Geometry: final body of the model. Coordinates: model frame, mm. A direction names the side the tool comes from. Give positions to 0.01 mm unless a question says otherwise; leave off trailing zeros. Loops run counter-clockwise (first coordinate to the right, second up) from the corner with the lowest first, then second, coordinate; pieces in that order, holes last. Notation, with made-up numbers: (7, 39.5) -> (28, 39.5) arc R21 ccw to (28, 53.5) -> close; hole circle Ø3 at (-8, -19.5). An arc over 180 degrees is marked (long way). One line per question, with ' | ' between items. Start each with the question number.
Item 1: Section D-D on x = 262.5. Return loops of the section in (y, z).
Item 2: Section C-C on x = -12. Return loops of the section in (y, z).
Item 3: Material intervals for line 1 along Y through (x, z) = (-311.95, 6); line 2 along Z through (x, y) = (312, -68); line 3 along Z through (x, y) = (-81, -12), sorted ascending. Write a range as [from, to].
Item 4: Set-up query: faces 4 (the flat face through (-326.8, -4.6, 0)), 5 (the flat face through (2, -17, 103)), 6 (the flat face through (-322, -61, 0)). Return all of +Z, -Z, +X, -X, +Y, -Y with unobstructed straight access to the full face (end or side cutting, diameter ignored); none if empty.
Item 5: Section A-A on y = -79.5. Return loops of the section in (x, z).
Item 6: Pin query (flat end, axial travel): P1, Ø0.5, axis at x = -312, y = -60, coming from the +Z side; P2, Ø3, axis at x = 110.3, z = 6, coming from the -Y side; P3, Ø9, axis at x = 71, z = 5.5, coming from the -Y side. Return the tip coordinate at first contact, or that it passes through.
Item 7: Mould query, pull axis X, two halves, no side actions, for faces 1 (the flat face through (4, 1, 51)), 2 (the flat face through (-4, 0, 51)), 3 (the cylindrical face through (-326.889, -3.563, 51.272)). Classes: released by +X, released by -X, zero draft, split by the parting line, or undercut.
Item 8: Section B-B on z = 18. Return loops of the section in (x, y), then the cut area to 3 significant figures.
from build123d import *

# Parameters (mm, degrees)
BASE_FLANGE1_DEPTH             = 104
EDGE_FLANGE1_STRIP_W           = 6
EDGE_FLANGE1_STRIP_H           = 1
EDGE_FLANGE1_STRIP_CUT_DEPTH   = 621.4
EDGE_FLANGE1_RELIEF_W          = 6.5
EDGE_FLANGE1_RELIEF_H          = 0.5
EDGE_FLANGE1_RELIEF_CUT_DEPTH  = 1
EDGE_FLANGE1_DEPTH             = 621.4
EDGE_FLANGE2_STRIP_W           = 6
EDGE_FLANGE2_STRIP_H           = 1
EDGE_FLANGE2_STRIP_CUT_DEPTH   = 621.4
EDGE_FLANGE2_DEPTH             = 621.4
EDGE_FLANGE3_STRIP_W           = 6
EDGE_FLANGE3_STRIP_H           = 1
EDGE_FLANGE3_STRIP_CUT_DEPTH   = 80
EDGE_FLANGE3_RELIEF_W          = 6.5
EDGE_FLANGE3_RELIEF_H          = 0.5
EDGE_FLANGE3_RELIEF_CUT_DEPTH  = 1
EDGE_FLANGE3_DEPTH             = 80
EDGE_FLANGE4_STRIP_W           = 6
EDGE_FLANGE4_STRIP_H           = 1
EDGE_FLANGE4_STRIP_CUT_DEPTH   = 80
EDGE_FLANGE4_DEPTH             = 80
EDGE_FLANGE5_STRIP_W           = 6
EDGE_FLANGE5_STRIP_H           = 1
EDGE_FLANGE5_STRIP_CUT_DEPTH   = 221.4
EDGE_FLANGE5_RELIEF_W          = 6.5
EDGE_FLANGE5_RELIEF_H          = 0.5
EDGE_FLANGE5_RELIEF_CUT_DEPTH  = 1
EDGE_FLANGE5_DEPTH             = 221.4
SKETCH22_R                     = 2.5
CUT_EXTRUDE1_DEPTH             = 1
SKETCH23_R                     = 2.5
CUT_EXTRUDE2_DEPTH             = 3
CUT_EXTRUDE2_DIRECTION_2_REACH = 661.378
EDGE_FLANGE6_STRIP_W           = 6
EDGE_FLANGE6_STRIP_H           = 1
EDGE_FLANGE6_STRIP_CUT_DEPTH   = 221.4
EDGE_FLANGE6_DEPTH             = 221.4
EDGE_FLANGE6_FLAT_DEPTH        = 1


# Sheet-metal steps are written as plain solids
with BuildPart() as part:
    # Sketch1 → Base-Flange1 (new body)
    with BuildSketch(Plane.XY):
        with BuildLine():
            Line((-330.7, -100), (-330.7, -15))
            ThreePointArc((-330.7, -15), (-326.306601718, -4.393398282), (-315.7, 0))
            Line((-315.7, 0), (315.7, 0))
            ThreePointArc((315.7, 0), (326.306601718, -4.393398282), (330.7, -15))
            Line((330.7, -15), (330.7, -100))
            Line((330.7, -100), (331.7, -100))
            Line((331.7, -100), (331.7, -15))
            ThreePointArc((331.7, -15), (327.013708499, -3.686291501), (315.7, 1))
            Line((315.7, 1), (-315.7, 1))
            ThreePointArc((-315.7, 1), (-327.013708499, -3.686291501), (-331.7, -15))
            Line((-331.7, -15), (-331.7, -100))
            Line((-331.7, -100), (-330.7, -100))
        make_face()
    extrude(amount=BASE_FLANGE1_DEPTH)

    # Edge-Flange1 strip (across the edge) → Edge-Flange1 strip cut (cut)
    with BuildSketch(Plane(origin=(-310.7, 0, 0), x_dir=(0, 0, 1), z_dir=(1, 0, 0))):
        with Locations((-2, -0.5)):
            Rectangle(EDGE_FLANGE1_STRIP_W, EDGE_FLANGE1_STRIP_H)
    extrude(amount=EDGE_FLANGE1_STRIP_CUT_DEPTH, mode=Mode.SUBTRACT)

    # Edge-Flange1 relief (on the sheet) → Edge-Flange1 relief cut (cut)
    with BuildSketch(Plane(origin=(-310.7, 0, 1), x_dir=(0, 0, 1), z_dir=(0, -1, 0))):
        with Locations((-2.75, 0.25)):
            Rectangle(EDGE_FLANGE1_RELIEF_W, EDGE_FLANGE1_RELIEF_H)
        with Locations((-2.75, -621.65)):
            Rectangle(EDGE_FLANGE1_RELIEF_W, EDGE_FLANGE1_RELIEF_H)
    extrude(amount=-EDGE_FLANGE1_RELIEF_CUT_DEPTH, mode=Mode.SUBTRACT)

    # Edge-Flange1 section (across the edge) → Edge-Flange1 (add)
    with BuildSketch(Plane(origin=(-310.7, 0, 0), x_dir=(0, 0, 1), z_dir=(1, 0, 0))):
        with BuildLine():
            Line((-1, 1), (-1, 19))
            Line((-1, 19), (0, 19))
            Line((0, 19), (0, 1))
            ThreePointArc((0, 1), (0.292893219, 0.292893219), (1, 0))
            Line((1, 0), (1, -1))
            ThreePointArc((1, -1), (-0.414213562, -0.414213562), (-1, 1))
        make_face()
    extrude(amount=EDGE_FLANGE1_DEPTH)

    # Edge-Flange2 strip (across the edge) → Edge-Flange2 strip cut (cut)
    with BuildSketch(Plane(origin=(-310.7, -19, 0), x_dir=(0, 1, 0), z_dir=(1, 0, 0))):
        with Locations((-1, -0.5)):
            Rectangle(EDGE_FLANGE2_STRIP_W, EDGE_FLANGE2_STRIP_H)
    extrude(amount=EDGE_FLANGE2_STRIP_CUT_DEPTH, mode=Mode.SUBTRACT)

    # Edge-Flange2 section (across the edge) → Edge-Flange2 (add)
    with BuildSketch(Plane(origin=(-310.7, -19, 0), x_dir=(0, 1, 0), z_dir=(1, 0, 0))):
        with BuildLine():
            Line((0, 1), (0, 12))
            Line((0, 12), (1, 12))
            Line((1, 12), (1, 1))
            ThreePointArc((1, 1), (1.292893219, 0.292893219), (2, 0))
            Line((2, 0), (2, -1))
            ThreePointArc((2, -1), (0.585786438, -0.414213562), (0, 1))
        make_face()
    extrude(amount=EDGE_FLANGE2_DEPTH)

    # Edge-Flange3 strip (across the edge) → Edge-Flange3 strip cut (cut)
    with BuildSketch(Plane(origin=(-330.7, -100, 0), x_dir=(0, 0, 1), z_dir=(0, 1, 0))):
        with Locations((-2, -0.5)):
            Rectangle(EDGE_FLANGE3_STRIP_W, EDGE_FLANGE3_STRIP_H)
    edge_flange3_strip_cut = extrude(amount=EDGE_FLANGE3_STRIP_CUT_DEPTH, mode=Mode.SUBTRACT)

    # Edge-Flange3 relief (on the sheet) → Edge-Flange3 relief cut (cut)
    with BuildSketch(Plane(origin=(-330.7, -100, 1), x_dir=(0, 0, 1), z_dir=(1, 0, 0))):
        with Locations((-2.75, -80.25)):
            Rectangle(EDGE_FLANGE3_RELIEF_W, EDGE_FLANGE3_RELIEF_H)
    edge_flange3_relief_cut = extrude(amount=-EDGE_FLANGE3_RELIEF_CUT_DEPTH, mode=Mode.SUBTRACT)

    # Edge-Flange3 section (across the edge) → Edge-Flange3 (add)
    with BuildSketch(Plane(origin=(-330.7, -100, 0), x_dir=(0, 0, 1), z_dir=(0, 1, 0))):
        with BuildLine():
            Line((-1, 1), (-1, 19))
            Line((-1, 19), (0, 19))
            Line((0, 19), (0, 1))
            ThreePointArc((0, 1), (0.292893219, 0.292893219), (1, 0))
            Line((1, 0), (1, -1))
            ThreePointArc((1, -1), (-0.414213562, -0.414213562), (-1, 1))
        make_face()
    edge_flange3 = extrude(amount=EDGE_FLANGE3_DEPTH)

    # Edge-Flange4 strip (across the edge) → Edge-Flange4 strip cut (cut)
    with BuildSketch(Plane(origin=(-311.7, -100, 0), x_dir=(-1, 0, 0), z_dir=(0, 1, 0))):
        with Locations((-1, -0.5)):
            Rectangle(EDGE_FLANGE4_STRIP_W, EDGE_FLANGE4_STRIP_H)
    edge_flange4_strip_cut = extrude(amount=EDGE_FLANGE4_STRIP_CUT_DEPTH, mode=Mode.SUBTRACT)

    # Edge-Flange4 section (across the edge) → Edge-Flange4 (add)
    with BuildSketch(Plane(origin=(-311.7, -100, 0), x_dir=(-1, 0, 0), z_dir=(0, 1, 0))):
        with BuildLine():
            Line((0, 1), (0, 12))
            Line((0, 12), (1, 12))
            Line((1, 12), (1, 1))
            ThreePointArc((1, 1), (1.292893219, 0.292893219), (2, 0))
            Line((2, 0), (2, -1))
            ThreePointArc((2, -1), (0.585786438, -0.414213562), (0, 1))
        make_face()
    edge_flange4 = extrude(amount=EDGE_FLANGE4_DEPTH)

    # Mirror1: Edge-Flange3 strip cut, Edge-Flange3 relief cut, Edge-Flange3, Edge-Flange4 strip cut, Edge-Flange4 across plane
    add(edge_flange3_strip_cut.mirror(Plane(origin=(0, 0, 0), x_dir=(0, 0, 1), z_dir=(1, 0, 0))), mode=Mode.SUBTRACT)
    add(edge_flange3_relief_cut.mirror(Plane(origin=(0, 0, 0), x_dir=(0, 0, 1), z_dir=(1, 0, 0))), mode=Mode.SUBTRACT)
    add(edge_flange3.mirror(Plane(origin=(0, 0, 0), x_dir=(0, 0, 1), z_dir=(1, 0, 0))))
    add(edge_flange4_strip_cut.mirror(Plane(origin=(0, 0, 0), x_dir=(0, 0, 1), z_dir=(1, 0, 0))), mode=Mode.SUBTRACT)
    add(edge_flange4.mirror(Plane(origin=(0, 0, 0), x_dir=(0, 0, 1), z_dir=(1, 0, 0))))

    # Edge-Flange5 strip (across the edge) → Edge-Flange5 strip cut (cut)
    with BuildSketch(Plane(origin=(110.7, 0, 104), x_dir=(0, 0, -1), z_dir=(-1, 0, 0))):
        with Locations((-1, -0.5)):
            Rectangle(EDGE_FLANGE5_STRIP_W, EDGE_FLANGE5_STRIP_H)
    extrude(amount=EDGE_FLANGE5_STRIP_CUT_DEPTH, mode=Mode.SUBTRACT)

    # Edge-Flange5 relief (on the sheet) → Edge-Flange5 relief cut (cut)
    with BuildSketch(Plane(origin=(110.7, 0, 102), x_dir=(0, 0, -1), z_dir=(0, -1, 0))):
        with Locations((-2.75, 0.25)):
            Rectangle(EDGE_FLANGE5_RELIEF_W, EDGE_FLANGE5_RELIEF_H)
        with Locations((-2.75, -221.65)):
            Rectangle(EDGE_FLANGE5_RELIEF_W, EDGE_FLANGE5_RELIEF_H)
    extrude(amount=-EDGE_FLANGE5_RELIEF_CUT_DEPTH, mode=Mode.SUBTRACT)

    # Edge-Flange5 section (across the edge) → Edge-Flange5 (add)
    with BuildSketch(Plane(origin=(110.7, 0, 104), x_dir=(0, 0, -1), z_dir=(-1, 0, 0))):
        with BuildLine():
            Line((0, 1), (0, 35.5))
            Line((0, 35.5), (1, 35.5))
            Line((1, 35.5), (1, 1))
            ThreePointArc((1, 1), (1.292893219, 0.292893219), (2, 0))
            Line((2, 0), (2, -1))
            ThreePointArc((2, -1), (0.585786438, -0.414213562), (0, 1))
        make_face()
    extrude(amount=EDGE_FLANGE5_DEPTH)

    # Sketch22 → Cut-Extrude1 (cut)
    with BuildSketch(Plane.XZ.offset(19)):
        with Locations(Location((-249.7, 6, 0), (0, 0, 270))):
            Circle(SKETCH22_R)
        with Locations(Location((-69.7, 6, 0), (0, 0, 270))):
            Circle(SKETCH22_R)
        with Locations(Location((110.3, 6, 0), (0, 0, 270))):
            Circle(SKETCH22_R)
        with Locations(Location((290.3, 6, 0), (0, 0, 270))):
            Circle(SKETCH22_R)
        with Locations((470.3, 6)):
            Circle(SKETCH22_R)
        with Locations((650.3, 6)):
            Circle(SKETCH22_R)
        with Locations((830.3, 6)):
            Circle(SKETCH22_R)
    extrude(amount=-CUT_EXTRUDE1_DEPTH, mode=Mode.SUBTRACT)

    # Sketch23 → Cut-Extrude2 (cut)
    with BuildSketch(Plane.ZY.offset(-311.7)):
        with Locations(Location((6, -68, 0), (0, 0, 180))):
            Circle(SKETCH23_R)
    extrude(amount=-CUT_EXTRUDE2_DEPTH, mode=Mode.SUBTRACT)

    # Cut-Extrude2 direction 2: up to this face of the body (flat: up to its plane)
    cut_extrude2_direction_2_end = Plane(part.part.faces().sort_by_distance((-312.7, -60, 6.5))[0])
    # Sketch23 → Cut-Extrude2 direction 2 (cut, up to the picked face)
    with BuildSketch(Plane.ZY.offset(-311.7), mode=Mode.PRIVATE) as cut_extrude2_direction_2_sk1:
        with Locations(Location((6, -68, 0), (0, 0, 180))):
            Circle(SKETCH23_R)
    cut_extrude2_direction_2_tool1 = split(extrude(cut_extrude2_direction_2_sk1.sketch, amount=CUT_EXTRUDE2_DIRECTION_2_REACH, mode=Mode.PRIVATE), bisect_by=cut_extrude2_direction_2_end, keep=Keep.BOTH, mode=Mode.PRIVATE)
    add(cut_extrude2_direction_2_tool1.solids().sort_by(Axis((311.7, -68, 6), (-1, 0, 0)))[0], mode=Mode.SUBTRACT)

    # Edge-Flange6 strip (across the edge) → Edge-Flange6 strip cut (cut)
    with BuildSketch(Plane(origin=(110.7, -35.5, 103), x_dir=(0, 1, 0), z_dir=(-1, 0, 0))):
        with Locations((-1, -0.5)):
            Rectangle(EDGE_FLANGE6_STRIP_W, EDGE_FLANGE6_STRIP_H)
    extrude(amount=EDGE_FLANGE6_STRIP_CUT_DEPTH, mode=Mode.SUBTRACT)

    # Edge-Flange6 bend section (across the edge) → Edge-Flange6 (add)
    with BuildSketch(Plane(origin=(110.7, -35.5, 103), x_dir=(0, 1, 0), z_dir=(-1, 0, 0))):
        with BuildLine():
            Line((0, 1), (1, 1))
            ThreePointArc((1, 1), (1.292893219, 0.292893219), (2, 0))
            Line((2, 0), (2, -1))
            ThreePointArc((2, -1), (0.585786438, -0.414213562), (0, 1))
        make_face()
    extrude(amount=EDGE_FLANGE6_DEPTH)

    # Edge-Flange6 profile (on flange) → Edge-Flange6 flat (add)
    with BuildSketch(Plane(origin=(0, -35.5, 103), x_dir=(1, 0, 0), z_dir=(0, 1, 0))):
        with BuildLine():
            Line((-110.7, 1), (110.7, 1))
            Line((110.7, 1), (110.7, 11))
            ThreePointArc((110.7, 11), (109.821320344, 13.121320344), (107.7, 14))
            Line((107.7, 14), (-107.7, 14))
            ThreePointArc((-107.7, 14), (-109.821320344, 13.121320344), (-110.7, 11))
            Line((-110.7, 11), (-110.7, 1))
        make_face()
    extrude(amount=EDGE_FLANGE6_FLAT_DEPTH)


solid = part.part
Result sheet:
1) outline: (-19, 1) arc R2 ccw to (-17, -1) -> (-1, -1) arc R2 ccw to (1, 1) -> (1, 104) -> (0, 104) -> (0, 1) arc R1 cw to (-1, 0) -> (-17, 0) arc R1 cw to (-18, 1) -> (-18, 12) -> (-19, 12) -> close
2) outline: (-35.5, 89) -> (-34.5, 89) -> (-34.5, 102) arc R1 cw to (-33.5, 103) -> (-1, 103) arc R1 cw to (0, 102) -> (0, 1) arc R1 cw to (-1, 0) -> (-17, 0) arc R1 cw to (-18, 1) -> (-18, 12) -> (-19, 12) -> (-19, 1) arc R2 ccw to (-17, -1) -> (-1, -1) arc R2 ccw to (1, 1) -> (1, 102) arc R2 ccw to (-1, 104) -> (-33.5, 104) arc R2 ccw to (-35.5, 102) -> close
3) line 1: y = [-100, -70.5], [-65.5, -20], [0, 1] | line 2: z = [-0.05, 3.5], [8.5, 12] | line 3: z = [-1, 0], [103, 104]
4) face 4: -Z, -X, +Y | face 5: none | face 6: +Z, -Y
5) outline: (-331.7, 1) arc R2 ccw to (-329.7, -1) -> (-313.7, -1) arc R2 ccw to (-311.7, 1) -> (-311.7, 12) -> (-312.7, 12) -> (-312.7, 1) arc R1 cw to (-313.7, 0) -> (-329.7, 0) arc R1 cw to (-330.7, 1) -> (-330.7, 104) -> (-331.7, 104) -> close; (311.7, 1) arc R2 ccw to (313.7, -1) -> (329.7, -1) arc R2 ccw to (331.7, 1) -> (331.7, 104) -> (330.7, 104) -> (330.7, 1) arc R1 cw to (329.7, 0) -> (313.7, 0) arc R1 cw to (312.7, 1) -> (312.7, 12) -> (311.7, 12) -> close
6) P1: stops at z = 12 | P2: stops at y = 0 | P3: stops at y = -19
7) face 1: zero draft | face 2: undercut | face 3: released by -X
8) outline: (-331.7, -100) -> (-330.7, -100) -> (-330.7, -15) arc R15 cw to (-315.7, 0) -> (315.7, 0) arc R15 cw to (330.7, -15) -> (330.7, -100) -> (331.7, -100) -> (331.7, -15) arc R16 ccw to (315.7, 1) -> (-315.7, 1) arc R16 ccw to (-331.7, -15) -> close | area: 850 mm²
